The listing builds one solid part. Answer for the finished solid, in the listing's coordinates (mm). Face numbers are marked on the shaded views. A direction names the side the tool comes from. Give positions to 0.01 mm unless a question says otherwise; leave off trailing zeros. Order: outer loops, then holes, each group sorted by start corner. A loop starts at its lowest first (then second) coordinate and runs counter-clockwise, first axis right, second up. Notation, with made-up numbers: (76.25, 5) - (122.25, 5) arc R21 cw to (122.25, 19) - close; hole circle Ø10 at (-14, 81.25). An arc over 180 degrees is marked (long way). Write each question's results on one line, items separated by ' | '. Start each with the question number.
1. Determine the mould class of the marked faces 3, 4, 5 and 6 for opening direction X: released by +X, released by -X, zero draft, split by the parting line, or undercut.
2. Which of the six approach directions +Z, -Z, +X, -X, +Y, -Y give full straight-line access (tool end or side, diameter ignored) to the marked faces 1 and 2?
3. Find the intervals of material crossed by L1, parallel to X at y = 96, z = 5.75; L2, parallel to Y at x = 7.5, z = 20; L3, parallel to Y at x = 15.5, z = 7.25, in increasing order.
4. Section B-B (y = 122) is taken. Give the vertices of the cut face in (x, z).
5. Flat-ended cylindrical pins translate along their axes: pin 1 (8 mm diameter, centred on x = 15, z = 15.5, fed in from +Y); pin 2 (3 mm diameter, centred on x = 6, z = 12, fed in from -Y); pin 3 (6.5 mm diameter, centred on x = 10, z = 16, fed in from -Y). Find the tip coordinate at first contact, or state that the pin passes through.
6. Section A-A (z = 9) is taken. Give the vertices of the cut face in (x, y).
from build123d import *

# Parameters (mm, degrees)
F1_DEPTH    = 25.4
F0_W        = 38.1
F0_H        = 76.2
F2_DEPTH    = 25.4
F3_T        = -2.54
F4_T1_DEPTH = 101.6
F4_T3_DEPTH = 50.8
F4_T5_DEPTH = 50.8
F4_T7_DEPTH = 63.5


# Not quite as in the source:
# - a fillet or chamfer that OpenCascade refuses, or shapes differently, is made with other operations: its cross-section is extruded or revolved along the edge and cut away or added


with BuildPart() as f1:
    # F0 (on Top) → F1 (new body)
    with BuildSketch(Plane.XY):
        Polygon((25.0072174214, -22.3877525396), (-13.0927825786, -22.3877525396), (5.9572174214, -39.1882733649), align=None)
    extrude(amount=F1_DEPTH)

    # F0 (on Top) → F2 (join)
    with BuildSketch(Plane.XY):
        with Locations((5.9572174214, 15.7122474604)):
            Rectangle(F0_W, F0_H)
    extrude(amount=F2_DEPTH)

    # F3
    f3_openings = [f1.faces().sort_by_distance(p)[0] for p in [
        (5.957217, 11.373102, 0),
    ]]
    offset(amount=F3_T, openings=f3_openings)

    # F4: fillet of radius 5.08 on 5 edges, made by hand

    # F4_s2 → F4_t1 (cut)
    with BuildSketch(Plane.XZ.offset(-66.5122474604)):
        with BuildLine():
            ThreePointArc((25.0072174214, 5.08), (23.5193198698, 1.4878975516), (19.9272174214, 0))
            Line((19.9272174214, 0), (25.0072174214, 0))
            Line((25.0072174214, 0), (25.0072174214, 5.08))
        make_face()
        with BuildLine():
            ThreePointArc((-13.0927825786, 5.08), (-11.604885027, 1.4878975516), (-8.0127825786, 0))
            Line((-8.0127825786, 0), (-13.0927825786, 0))
            Line((-13.0927825786, 0), (-13.0927825786, 5.08))
        make_face()
    extrude(amount=F4_T1_DEPTH, mode=Mode.SUBTRACT)

    # F4_s4 → F4_t3 (cut)
    with BuildSketch(Plane(origin=(-25.6145200068, -22.5898832967, 0), x_dir=(0, 0, 1), z_dir=(0.75, 0.6614378278, 0))):
        with BuildLine():
            ThreePointArc((5.08, 33.3315339744), (1.4878975516, 31.8436364228), (0, 28.2515339744))
            Line((0, 28.2515339744), (0, 33.3315339744))
            Line((0, 33.3315339744), (5.08, 33.3315339744))
        make_face()
    extrude(amount=F4_T3_DEPTH, mode=Mode.SUBTRACT)

    # F4_s6 → F4_t5 (cut)
    with BuildSketch(Plane(origin=(-5.7836103942, 5.1006649277, 0), x_dir=(0, 0, 1), z_dir=(0.75, -0.6614378278, 0))):
        with BuildLine():
            ThreePointArc((5.08, 25.4508760729), (1.4878975516, 23.9629785214), (0, 20.3708760729))
            Line((0, 20.3708760729), (0, 25.4508760729))
            Line((0, 25.4508760729), (5.08, 25.4508760729))
        make_face()
    extrude(amount=F4_T5_DEPTH, mode=Mode.SUBTRACT)

    # F4_s8 → F4_t7 (cut)
    with BuildSketch(Plane.YZ.offset(-25.7927825786)):
        with BuildLine():
            ThreePointArc((53.8122474604, 5.08), (52.3243499088, 1.4878975516), (48.7322474604, 0))
            Line((48.7322474604, 0), (53.8122474604, 0))
            Line((53.8122474604, 0), (53.8122474604, 5.08))
        make_face()
    extrude(amount=F4_T7_DEPTH, mode=Mode.SUBTRACT)

    # F5: F1 across face


with BuildPart() as f1_1:
    add(f1.part)
    add(f1.part.mirror(Plane(origin=(5.9572174214, 53.8122474604, 15.24), x_dir=(-1, 0, 0), z_dir=(0, 1, 0))))


solid = f1_1.part
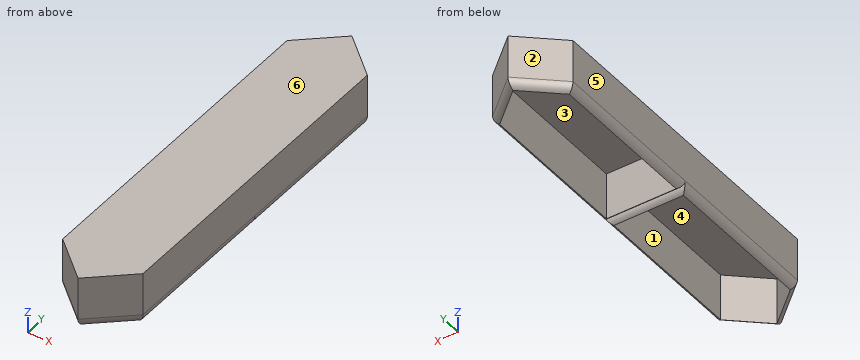
Reported:
1) face 3: undercut | face 4: undercut | face 5: released by -X | face 6: zero draft
2) face 1: -Z | face 2: +Z, -Z, -X, +Y
3) L1: -13.09 to -10.55, 22.47 to 25.01 | L2: -37.83 to -34.44, 51.27 to 56.35, 142.07 to 145.45 | L3: -30.77 to -27.39, 51.27 to 56.35, 135.01 to 138.4
4) outline: (-13.09, 5.08) arc R5.08 ccw to (-10.55, 0.68) - (-10.55, 22.86) - (22.47, 22.86) - (22.47, 0.68) arc R5.08 ccw to (25.01, 5.08) - (25.01, 25.4) - (-13.09, 25.4) - close
5) pin 1: y = 142.37 | pin 2: y = -39.19 | pin 3: y = -38.49
6) outline: (-13.09, -22.39) - (5.96, -39.19) - (25.01, -22.39) - (25.01, 130.01) - (5.96, 146.81) - (-13.09, 130.01) - close; hole (-10.55, -21.24) - (5.96, -35.8) - (22.47, -21.24) - (22.47, 51.27) - (-10.55, 51.27) - close; hole (-10.55, 56.35) - (22.47, 56.35) - (22.47, 128.87) - (5.96, 143.43) - (-10.55, 128.87) - close
